```python
from build123d import *

# Parameters (mm, degrees)
SKETCH1_R               = 37.5
SKETCH1_R_2             = 1.7
BOSS_EXTRUDE1_DEPTH     = 20
CUT_EXTRUDE1_DEPTH      = 57.678920244
CUT_EXTRUDE1_DEPTH_BACK = 57.678920244
SKETCH2_W               = 10.2
SKETCH2_H               = 10.2
CUT_EXTRUDE2_START      = -10
SKETCH3_R               = 1.7
CUT_EXTRUDE2_DEPTH      = 10
CUT_EXTRUDE4_START      = -10
SKETCH4_W               = 10.71
SKETCH4_H               = 10.2
CUT_EXTRUDE4_DEPTH      = 10
BOSS_EXTRUDE2_START     = 8
BOSS_EXTRUDE2_DEPTH     = 5
SKETCH7_R               = 3
CUT_EXTRUDE5_DEPTH      = 5
SKETCH8_R               = 1.7
CUT_EXTRUDE6_DEPTH      = 15
FILLET1_R               = 5
SKETCH9_R               = 37.5
CUT_EXTRUDE7_DEPTH      = 2
CUT_EXTRUDE8_START      = -10
CUT_EXTRUDE8_DEPTH      = 10
FILLET3_R               = 7.5


with BuildPart() as part:
    # Sketch1 → Boss-Extrude1 (new body)
    with BuildSketch(Plane(origin=(0, 0, 0), x_dir=(0, 0, -1), z_dir=(1, 0, 0))):
        Circle(SKETCH1_R)
        with Locations((0, 27)):
            Circle(SKETCH1_R_2, mode=Mode.SUBTRACT)
        with Locations((23.382685902, -13.5)):
            Circle(SKETCH1_R_2, mode=Mode.SUBTRACT)
        with Locations((-23.382685902, -13.5)):
            Circle(SKETCH1_R_2, mode=Mode.SUBTRACT)
    extrude(amount=BOSS_EXTRUDE1_DEPTH)

    # Sketch2 → Cut-Extrude1 (cut, two sides: drawn at the far end of the back side and taken through both)
    with BuildSketch(Plane.XY.offset(-CUT_EXTRUDE1_DEPTH_BACK)):
        with Locations((10, 0)):
            Rectangle(SKETCH2_W, SKETCH2_H)
    extrude(amount=CUT_EXTRUDE1_DEPTH + CUT_EXTRUDE1_DEPTH_BACK, mode=Mode.SUBTRACT)

    # Sketch3 → Cut-Extrude2 (cut)
    # profile 1 of 2: a face of its own
    with BuildSketch(Plane(origin=(20, 0, 0), x_dir=(0, 0, -1), z_dir=(1, 0, 0)).offset(CUT_EXTRUDE2_START)):
        with BuildLine():
            Line((-36.11426311, 10.1), (36.11426311, 10.1))
            ThreePointArc((36.11426311, 10.1), (0, 37.5), (-36.11426311, 10.1))
        make_face()
        with Locations((0, 27)):
            Circle(SKETCH3_R, mode=Mode.SUBTRACT)
    # profile 2 of 2: a face of its own
    with BuildSketch(Plane(origin=(20, 0, 0), x_dir=(0, 0, -1), z_dir=(1, 0, 0)).offset(CUT_EXTRUDE2_START)):
        with BuildLine():
            ThreePointArc((-36.11426311, -10.1), (0, -37.5), (36.11426311, -10.1))
            Line((36.11426311, -10.1), (-36.11426311, -10.1))
        make_face()
        with Locations((-23.382685902, -13.5)):
            Circle(SKETCH3_R, mode=Mode.SUBTRACT)
        with Locations((23.382685902, -13.5)):
            Circle(SKETCH3_R, mode=Mode.SUBTRACT)
    extrude(amount=CUT_EXTRUDE2_DEPTH, mode=Mode.SUBTRACT)

    # Sketch4 → Cut-Extrude4 (cut)
    with BuildSketch(Plane(origin=(20, 0, 0), x_dir=(0, 0, -1), z_dir=(1, 0, 0)).offset(CUT_EXTRUDE4_START)):
        with BuildLine():
            Line((-26.79, -5.1), (-26.79, 5.1))
            Line((-26.79, 5.1), (-37.151581393, 5.1))
            ThreePointArc((-37.151581393, 5.1), (-37.5, 0), (-37.151581393, -5.1))
            Line((-37.151581393, -5.1), (-26.79, -5.1))
        make_face()
        with Locations((-10.725, 0)):
            Rectangle(SKETCH4_W, SKETCH4_H)
        with Locations((10.695, 0)):
            Rectangle(SKETCH4_W, SKETCH4_H)
        with BuildLine():
            Line((37.151581393, 5.1), (26.76, 5.1))
            Line((26.76, 5.1), (26.76, -5.1))
            Line((26.76, -5.1), (37.151581393, -5.1))
            ThreePointArc((37.151581393, -5.1), (37.5, 0), (37.151581393, 5.1))
        make_face()
    extrude(amount=CUT_EXTRUDE4_DEPTH, mode=Mode.SUBTRACT)

    # Sketch6 → Boss-Extrude2 (add)
    with BuildSketch(Plane.XY.offset(BOSS_EXTRUDE2_START)):
        Polygon((20, 10.1), (10, 20.1), (10, 10.1), align=None)
        Polygon((10, -20.1), (10, -10.1), (20, -10.1), align=None)
    boss_extrude2 = extrude(amount=BOSS_EXTRUDE2_DEPTH)

    # Mirror1: Boss-Extrude2 across plane
    add(boss_extrude2.mirror(Plane.XY))

    # Sketch7 → Cut-Extrude5 (cut)
    with BuildSketch(Plane.ZY):
        with Locations((23.382685902, 13.5)):
            Circle(SKETCH7_R)
        with Locations((0, -27)):
            Circle(SKETCH7_R)
        with Locations((-23.382685902, 13.5)):
            Circle(SKETCH7_R)
    extrude(amount=-CUT_EXTRUDE5_DEPTH, mode=Mode.SUBTRACT)

    # Sketch8 → Cut-Extrude6 (cut)
    with BuildSketch(Plane.ZY):
        with Locations((-23.382685902, 13.5)):
            Circle(SKETCH8_R)
        with Locations((23.382685902, 13.5)):
            Circle(SKETCH8_R)
        with Locations((0, -27)):
            Circle(SKETCH8_R)
    extrude(amount=-CUT_EXTRUDE6_DEPTH, mode=Mode.SUBTRACT)

    # Fillet1
    fillet1_edges = [part.edges().sort_by_distance(p)[0] for p in [
        (20, 7.617677291, 36.718128938),
        (20, -7.617677291, -36.718128938),
        (20, 7.617677291, -36.718128938),
        (20, -7.617677291, 36.718128938),
    ]]
    fillet(fillet1_edges, radius=FILLET1_R)

    # Sketch9 → Cut-Extrude7 (cut)
    with BuildSketch(Plane.ZY):
        Circle(SKETCH9_R)
    extrude(amount=-CUT_EXTRUDE7_DEPTH, mode=Mode.SUBTRACT)

    # Sketch10 → Cut-Extrude8 (cut)
    with BuildSketch(Plane(origin=(10, 0, 0), x_dir=(0, 0, -1), z_dir=(1, 0, 0)).offset(CUT_EXTRUDE8_START)):
        with BuildLine():
            ThreePointArc((-10, 36.142080737), (-21.885509272, 30.451181979), (-31.068472766, 21))
            Line((-31.068472766, 21), (-10, 21))
            Line((-10, 21), (-10, 36.142080737))
        make_face()
        with BuildLine():
            Line((10, 21), (31.068472766, 21))
            ThreePointArc((31.068472766, 21), (21.885509272, 30.451181979), (10, 36.142080737))
            Line((10, 36.142080737), (10, 21))
        make_face()
        with BuildLine():
            Line((31.068472766, -21), (-31.068472766, -21))
            ThreePointArc((-31.068472766, -21), (0, -37.5), (31.068472766, -21))
        make_face()
    extrude(amount=CUT_EXTRUDE8_DEPTH, mode=Mode.SUBTRACT)

    # Fillet3
    fillet3_edges = [part.edges().sort_by_distance(p)[0] for p in [
        (6, -21, 31.068472766),
        (6, -21, -31.068472766),
        (6, 36.142080737, -10),
        (6, 21, -31.068472766),
        (6, 21, -10),
        (6, 36.142080737, 10),
        (6, 21, 10),
        (6, 21, 31.068472766),
    ]]
    fillet(fillet3_edges, radius=FILLET3_R)


solid = part.part
```
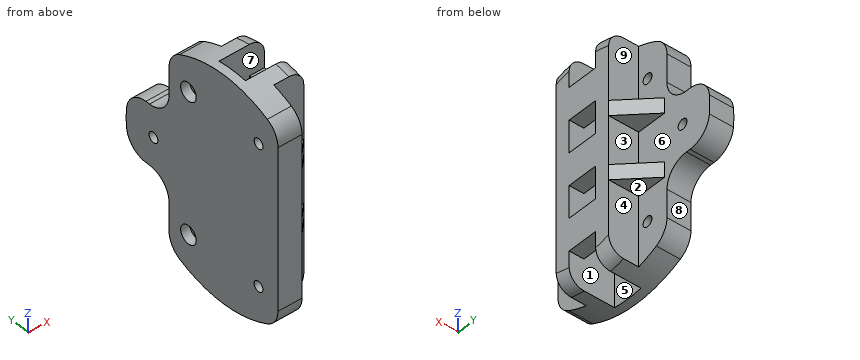
The listing builds one solid part. Answer for the finished solid, in the listing's coordinates (mm). Face numbers are marked on the shaded views. A direction names the side the tool comes from. Coordinates: 2 decimals unless noted, no trailing zeros. Write each loop counter-clockwise with the first axis right and the second up, starting at its lowest first coordinate (ties: lowest second). Pieces come first, ordered by that corner, then holes.
Q1. Find the intervals of material crossed by line 1 along Y through (x, z) = (18, -31.5); line 2 along Z through (x, y) = (12, -10.5); line 3 along Y through (x, z) = (5.5, 0), in increasing order.
Returned:
line 1: y = -10.1 to -5.1, 5.1 to 10.1
line 2: z = -13 to -8, 8 to 13
line 3: y = -21 to -5.1, 5.1 to 25.3, 28.7 to 37.5
Q2. Section D-D, the plane y = 13.5 is taken. Write down the section's boundary in (x, z), then the cut area to 3 significant figures.
Returned:
outline: (2, -34.99) - (10, -34.99) - (10, -25.08) - (5, -25.08) - (5, -26.38) - (2, -26.38) - close; (2, -20.38) - (5, -20.38) - (5, -21.68) - (10, -21.68) - (10, -13) - (16.6, -13) - (16.6, -8) - (10, -8) - (10, 8) - (16.6, 8) - (16.6, 13) - (10, 13) - (10, 21.68) - (5, 21.68) - (5, 20.38) - (2, 20.38) - close; (2, 26.38) - (5, 26.38) - (5, 25.08) - (10, 25.08) - (10, 34.99) - (2, 34.99) - close
area: 556 mm2
Q3. Section B-B, the plane x = 11.25 is taken. Write down the section's boundary in (y, z), then the cut area to 3 significant figures.
Returned:
outline: (-18.85, -13) - (-10.1, -13) - (-10.1, -36.11) arc R37.5 ccw to (-5.1, -37.15) - (-5.1, 37.15) arc R37.5 ccw to (-10.1, 36.11) - (-10.1, 13) - (-18.85, 13) - (-18.85, 8) - (-10.1, 8) - (-10.1, -8) - (-18.85, -8) - close; (5.1, -37.15) arc R37.5 ccw to (10.1, -36.11) - (10.1, -13) - (18.85, -13) - (18.85, -8) - (10.1, -8) - (10.1, 8) - (18.85, 8) - (18.85, 13) - (10.1, 13) - (10.1, 36.11) arc R37.5 ccw to (5.1, 37.15) - close
area: 909 mm2
Q4. Section A-A, the plane z = 0 is taken. Write down the section's boundary in (x, y).
Returned:
outline: (2, -21) - (10, -21) - (10, -10.1) - (20, -10.1) - (20, 10.1) - (10, 10.1) - (10, 25.3) - (2, 25.3) - close; (2, 28.7) - (10, 28.7) - (10, 37.5) - (2, 37.5) - close; hole (4.9, -5.1) - (15.1, -5.1) - (15.1, 5.1) - (4.9, 5.1) - close
Q5. Which of the six approach directions +Z, -Z, +X, -X, +Y, -Y give full straight-line access (tool end or side, diameter ignored) to the marked faces 5, 6, 7, 8 and 9?
Returned:
face 5: +Z, -Z
face 6: +X, +Y
face 7: none
face 8: -Z, +X, -X, +Y
face 9: +Z, +X, +Y
Q6. Section C-C, the plane y = -1 is taken. Write down the section's boundary in (x, z).
Returned:
outline: (2, -37.49) - (4.9, -37.49) - (4.9, 37.49) - (2, 37.49) - close; (15.1, -26.76) - (20, -26.76) - (20, -16.05) - (15.1, -16.05) - close; (15.1, -5.34) - (20, -5.34) - (20, 5.37) - (15.1, 5.37) - close; (15.1, 16.08) - (20, 16.08) - (20, 26.79) - (15.1, 26.79) - close
Q7. Given P1, Ø8, axis at x = 4.5, y = 20, coming from the -Z side; P2, Ø1.8, axis at y = 12.5, z = 22.5, coming from the -X side; P3, Ø8, axis at x = 17, y = 17.5, coming from the +Z side, each flat-ended and moving along its own axis, determine where each tip first touches the part or whether it passes through.
Returned:
P1: stops at z = -33.92
P2: stops at x = 5
P3: stops at z = 13
Q8. The mould has two halves that part along Z. Classify the marked faces 1, 2, 3 and 4: released by +Z, released by -Z, zero draft, split by the parting line, or undercut.
Returned:
face 1: undercut
face 2: released by -Z
face 3: undercut
face 4: zero draft
